```python
from build123d import *

# Parameters (mm, degrees)
F1_DEPTH = 57.15
F2_R     = 2.8624183912
F2_R_2   = 1.905
F3_DEPTH = 3.175
F4_R     = 1.905
F5_DEPTH = 3.175


with BuildPart() as f1:
    # F0 (on Top) → F1 (new body)
    with BuildSketch(Plane.XY):
        Polygon((-190.5, 0), (-190.5, -63.5), (63.5, -63.5), (63.5, 190.5), (0, 190.5), (0, 0), align=None)
    extrude(amount=F1_DEPTH)

    # F2 (on face) → F3 (join)
    with BuildSketch(Plane(origin=(0, 0, 0), x_dir=(1, 0, 0), z_dir=(0, 0, -1))):
        Polygon((-168.275, -3.175), (-28.575, -3.175), (-28.575, -28.575), (-3.175, -28.575), (-3.175, -168.275), (-28.575, -168.275), (-28.575, -193.675), (-3.175, -193.675), (66.675, -193.675), (92.075, -193.675), (92.075, -168.275), (66.675, -168.275), (66.675, 66.675), (-168.275, 66.675), (-168.275, 92.075), (-193.675, 92.075), (-193.675, 66.675), (-193.675, -3.175), (-193.675, -28.575), (-168.275, -28.575), align=None)
        Polygon((-190.5, 0), (-190.5, 63.5), (63.5, 63.5), (63.5, -190.5), (0, -190.5), (0, 0), align=None, mode=Mode.SUBTRACT)
        with Locations((-15.875, -180.975)):
            Circle(F2_R, mode=Mode.SUBTRACT)
        with Locations((79.375, -180.975)):
            Circle(F2_R_2, mode=Mode.SUBTRACT)
        with Locations((-180.975, -15.875)):
            Circle(F2_R_2, mode=Mode.SUBTRACT)
        with Locations((-180.975, 79.375)):
            Circle(F2_R_2, mode=Mode.SUBTRACT)
        with Locations((-15.875, -15.875)):
            Circle(F2_R_2, mode=Mode.SUBTRACT)
        Polygon((63.5, 63.5), (-190.5, 63.5), (-190.5, 0), (0, 0), (0, -190.5), (63.5, -190.5), align=None)
    extrude(amount=F3_DEPTH)

    # F4 (on face) → F5 (join)
    with BuildSketch(Plane.XY.offset(57.15)):
        Polygon((-28.575, 168.275), (-3.175, 168.275), (-3.175, 28.575), (-28.575, 28.575), (-28.575, 3.175), (-168.275, 3.175), (-168.275, 28.575), (-193.675, 28.575), (-193.675, 3.175), (-193.675, -66.675), (-193.675, -92.075), (-168.275, -92.075), (-168.275, -66.675), (66.675, -66.675), (66.675, 168.275), (92.075, 168.275), (92.075, 193.675), (66.675, 193.675), (-3.175, 193.675), (-28.575, 193.675), align=None)
        with Locations((-180.975, -79.375)):
            Circle(F4_R, mode=Mode.SUBTRACT)
        with Locations((-180.975, 15.875)):
            Circle(F4_R, mode=Mode.SUBTRACT)
        with Locations((-15.875, 15.875)):
            Circle(F4_R, mode=Mode.SUBTRACT)
        with Locations((-15.875, 180.975)):
            Circle(F4_R, mode=Mode.SUBTRACT)
        with Locations((79.375, 180.975)):
            Circle(F4_R, mode=Mode.SUBTRACT)
    extrude(amount=F5_DEPTH)


solid = f1.part
```
For this review, take the finished solid that the model builds, in its own axes (mm). A direction names the side the tool comes from. Coordinates: 2 decimals unless noted, no trailing zeros. Loops run counter-clockwise (first coordinate to the right, second up) from the corner with the lowest first, then second, coordinate; pieces in that order, holes last. Notation, with made-up numbers: (48.5, 86) -> (101.5, 86) arc R19 ccw to (101.5, 106) -> close; hole circle Ø2 at (37, -37.5). An arc over 180 degrees is marked (long way). Return JSON: item names as keys, results as strings. Group by question number.
(1) To check wall thickness, follow L1, parallel to Z at x = 64, y = 95.5 (3 decimals); L2, parallel to X at y = -30.5, z = 41.5; L3, parallel to Y at x = -84.5, z = 1.5. State the ranges of each line that lie inside material, in increasing order.
(2) For pin 1 Ø8 at (y, z) = (-25, 52) entering from +X; pin 2 Ø3 at (x, z) = (-156, 32) entering from +Y; pin 3 Ø6 at (x, z) = (49, 26) entering from -Y; pin 4 Ø6 at (x, y) = (-15.875, 15.875) entering from +Z (3 decimals), all flat-tipped, find the tip position at first contact; note any pin that passes through.
(3) Consider section A-A, the plane x = 72. Give the boundary of the cut face in (y, z) (3 decimals).
(4) Consider section B-B, the plane y = -4. Give the boundary of the cut face in (x, z) (3 decimals).
(5) Mouldability with a two-part tool opening along Z and no side actions: class faces 4 (the flat face through (-21, 21, 60.325)), 5 (the flat face through (-20, 18, 0)), 6 (the flat face through (-21, 17, -3.175)) as pulls with the +Z half, pulls with the -Z half, needs draft (parallel to the pull), parting line crosses it, or undercut.
(6) Tool access review of faces 1 (the flat face through (-65, -63.5, 28)), 2 (the flat face through (-20, 20, 57.15)), 3 (the flat face through (63.5, 62, 28)): name each direction out of +Z, -Z, +X, -X, +Y, -Y from which nothing blocks a thin tool from reaching the whole face with its end or side.
(7) Consider section C-C, the plane z = 11. Give the boundary of the cut face in (x, y), plus the area to 3 significant figures.
(8) Consider section D-D, the plane x = -137. Give the boundary of the cut face in (y, z) (3 decimals).
Results below:
{
 "1": {"L1": "z = -3.175 to 0, 57.15 to 60.325", "L2": "x = -190.5 to 63.5", "L3": "y = -63.5 to 0"},
 "2": {"pin 1": "stops at x = 63.5", "pin 2": "stops at y = 0", "pin 3": "stops at y = -63.5", "pin 4": "stops at z = 60.325"},
 "3": {"outline": "(168.275, -3.175) -> (193.675, -3.175) -> (193.675, 0) -> (168.275, 0) -> close; (168.275, 57.15) -> (193.675, 57.15) -> (193.675, 60.325) -> (168.275, 60.325) -> close"},
 "4": {"outline": "(-193.675, -3.175) -> (66.675, -3.175) -> (66.675, 0) -> (63.5, 0) -> (63.5, 57.15) -> (66.675, 57.15) -> (66.675, 60.325) -> (-193.675, 60.325) -> (-193.675, 57.15) -> (-190.5, 57.15) -> (-190.5, 0) -> (-193.675, 0) -> close"},
 "5": {"face 4": "pulls with the +Z half", "face 5": "undercut", "face 6": "pulls with the -Z half"},
 "6": {"face 1": "+X, -X, -Y", "face 2": "none", "face 3": "+X, +Y, -Y"},
 "7": {"outline": "(-190.5, -63.5) -> (63.5, -63.5) -> (63.5, 190.5) -> (0, 190.5) -> (0, 0) -> (-190.5, 0) -> close", "area": "28,200 mm2"},
 "8": {"outline": "(-66.675, -3.175) -> (3.175, -3.175) -> (3.175, 0) -> (0, 0) -> (0, 57.15) -> (3.175, 57.15) -> (3.175, 60.325) -> (-66.675, 60.325) -> (-66.675, 57.15) -> (-63.5, 57.15) -> (-63.5, 0) -> (-66.675, 0) -> close"}
}
